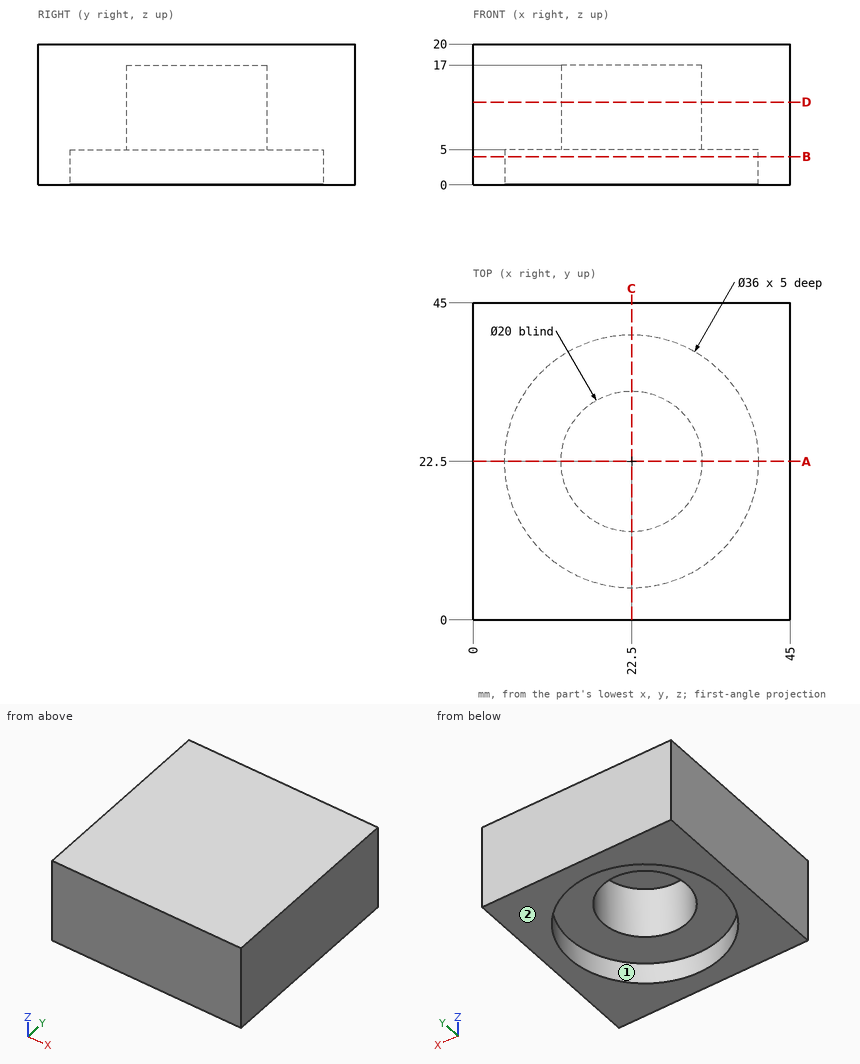
Here's the drawing with two shaded views (mm, measured from the low corner). I have some questions. A direction names the side the tool comes from. Give positions to 0.01 mm unless a question says otherwise; leave off trailing zeros. Loops run counter-clockwise (first coordinate to the right, second up) from the corner with the lowest first, then second, coordinate; pieces in that order, holes last. Notation, with made-up numbers: M 48,-33.75 L 82,-33.75 A30 cw 82,-8.75 Z; hole C -14,23.25 d4. An arc over 180 degrees is marked long. One line per item, written item: value.
(1) Suppose I cut it at B-B on z = 4. List the corners of the cut face in (x, y) for me.
Returned:
outline: M 0,0 L 45,0 L 45,45 L 0,45 Z; hole C 22.5,22.5 d36
(2) Suppose I cut it at D-D on z = 11.75. List the corners of the cut face in (x, y) for me.
Returned:
outline: M 0,0 L 45,0 L 45,45 L 0,45 Z; hole C 22.5,22.5 d20
(3) I need wall thicknesses on line 1 (Y direction, x = 22.5, z = 1.6); line 2 (Y direction, x = 22.5, z = 11.5). Which ranges of each line are inside material? Lowest first, please.
Returned:
line 1: 0 to 4.5, 40.5 to 45
line 2: 0 to 12.5, 32.5 to 45
(4) Will these pins go through, and if not, where does the flat tip stop? pin 1 (18 mm diameter, centred on x = 22.5, y = 22.5, fed in from -Z); pin 2 (22 mm diameter, centred on x = 25, y = 18.5, fed in from -Z).
Returned:
pin 1: z = 17
pin 2: z = 5
(5) Suppose I cut it at A-A on y = 22.5. List the corners of the cut face in (x, z) for me.
Returned:
outline: M 0,0 L 4.5,0 L 4.5,5 L 12.5,5 L 12.5,17 L 32.5,17 L 32.5,5 L 40.5,5 L 40.5,0 L 45,0 L 45,20 L 0,20 Z
(6) Which directions (+Z, -Z, +X, -X, +Y, -Y) give clear straight access to the entire face, cutting with the end or side of a thin tool? Please do the marked faces 1 and 2.
Returned:
face 1: -Z
face 2: -Z, +X, -X, +Y, -Y
